Drawing for the job (mm, zero at the part's lowest x, y, z). Round coordinates to 2 decimals unless told otherwise and drop trailing zeros. Write each loop counter-clockwise with the first axis right and the second up, starting at its lowest first coordinate (ties: lowest second). Pieces come first, ordered by that corner, then holes.
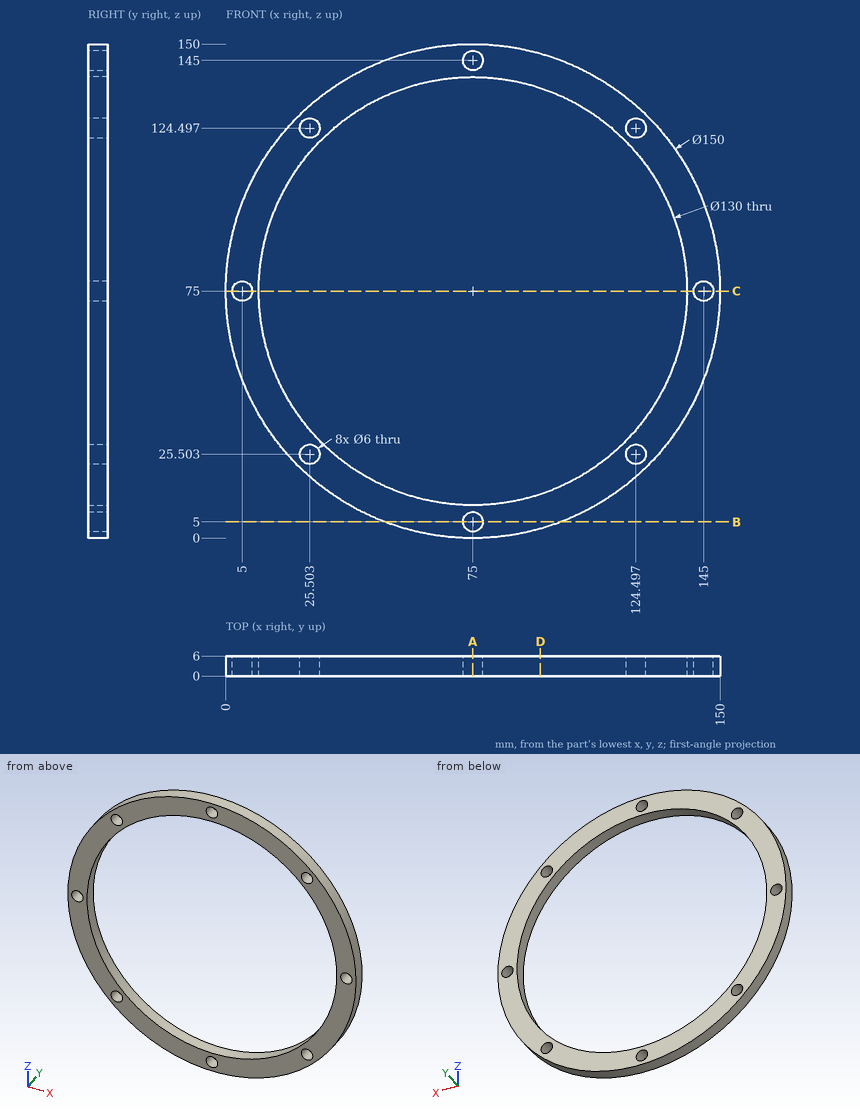
1) Cut at A-A on x = 75. List the corners of the cut face in (y, z).
2) Wall check: probe 1 along X at (y, z) = (3.7, 75); probe 2 along X at (y, z) = (3.3, 26) (1 decimal). Give the ranges that are in metal, low to high.
3) Cut at B-B on z = 5. List the corners of the cut face in (x, y) (1 decimal), and give its area (3 significant figures).
4) Cut at C-C on z = 75. List the corners of the cut face in (x, y).
5) Cut at D-D on x = 95.5. List the corners of the cut face in (y, z).
6) Flat gauge pins, fed straight in: pin 1 Ø8 at (x, z) = (145, 75) entering from -Y; pin 2 Ø1 at (x, y) = (29, 4) entering from -Z. Where does each tip first touch, or does it go through?
Result sheet:
1. outline: (0, 0) - (6, 0) - (6, 2) - (0, 2) - close; (0, 8) - (6, 8) - (6, 10) - (0, 10) - close; (0, 140) - (6, 140) - (6, 142) - (0, 142) - close; (0, 148) - (6, 148) - (6, 150) - (0, 150) - close
2. probe 1: x = 0 to 2, 8 to 10, 140 to 142, 148 to 150
2. probe 2: x = 18.2 to 22.5, 28.5 to 32.3, 117.7 to 121.5, 127.5 to 131.8
3. outline: (48.1, 0) - (72, 0) - (72, 6) - (48.1, 6) - close; (78, 0) - (101.9, 0) - (101.9, 6) - (78, 6) - close
3. area: 287 mm2
4. outline: (0, 0) - (2, 0) - (2, 6) - (0, 6) - close; (8, 0) - (10, 0) - (10, 6) - (8, 6) - close; (140, 0) - (142, 0) - (142, 6) - (140, 6) - close; (148, 0) - (150, 0) - (150, 6) - (148, 6) - close
5. outline: (0, 2.86) - (6, 2.86) - (6, 13.32) - (0, 13.32) - close; (0, 136.68) - (6, 136.68) - (6, 147.14) - (0, 147.14) - close
6. pin 1: stops at y = 0
6. pin 2: stops at z = 15.38
